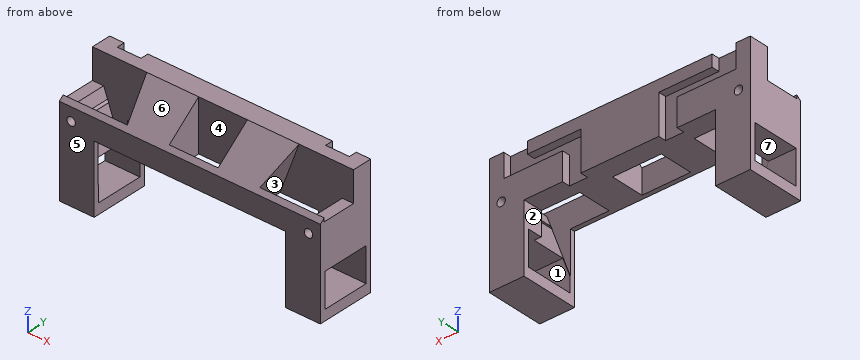
from build123d import *

# Parameters (mm, degrees)
CROQUIS1_W                  = 99
CROQUIS1_H                  = 49
SALIENTE_EXTRUIR1_DEPTH     = 22
CROQUIS2_W                  = 13
CROQUIS2_H                  = 18
CORTAR_EXTRUIR1_DEPTH       = 105.895766214
CROQUIS3_W                  = 3.5
CROQUIS3_H                  = 22
CORTAR_EXTRUIR2_DEPTH       = 105.895766214
CROQUIS4_W                  = 72.6
CROQUIS4_H                  = 26
CORTAR_EXTRUIR3_DEPTH       = 69.17620423
CORTAR_EXTRUIR4_DEPTH       = 79.584079892
CROQUIS7_W                  = 20.634922244
CROQUIS7_H                  = 12.8
CORTAR_EXTRUIR7_DEPTH       = 60
CROQUIS12_W                 = 20.6
CROQUIS12_H                 = 12.8
CORTAR_EXTRUIR8_DEPTH       = 60
CORTAR_EXTRUIR9_DEPTH       = 105.056653851
CORTAR_EXTRUIR9_DEPTH_BACK  = 105.056653851
CROQUIS16_W                 = 11.5
CROQUIS16_H                 = 12.8
CORTAR_EXTRUIR11_DEPTH      = 10
CROQUIS17_W                 = 11.5
CROQUIS17_H                 = 12.8
CORTAR_EXTRUIR12_DEPTH      = 10
CORTAR_EXTRUIR13_DEPTH      = 3
CORTAR_EXTRUIR14_DEPTH      = 69.17620423
CORTAR_EXTRUIR14_DEPTH_BACK = 69.17620423
CROQUIS20_R                 = 1.6


with BuildPart() as part:
    # Croquis1 → Saliente-Extruir1 (new body)
    with BuildSketch(Plane(origin=(0, 0, 0), x_dir=(1, 0, 0), z_dir=(0, 1, 0))):
        with Locations((10.676470588, -2.297794118)):
            Rectangle(CROQUIS1_W, CROQUIS1_H)
    extrude(amount=SALIENTE_EXTRUIR1_DEPTH)

    # Croquis2 → Cortar-Extruir1 (cut, through all)
    with BuildSketch(Plane.ZY.offset(38.823529412)):
        with Locations((-11.702205882, 11)):
            Rectangle(CROQUIS2_W, CROQUIS2_H)
    extrude(amount=-CORTAR_EXTRUIR1_DEPTH, mode=Mode.SUBTRACT)

    # Croquis3 → Cortar-Extruir2 (cut, through all)
    with BuildSketch(Plane.ZY.offset(38.823529412)):
        with Locations((25.047794118, 11)):
            Rectangle(CROQUIS3_W, CROQUIS3_H)
    extrude(amount=-CORTAR_EXTRUIR2_DEPTH, mode=Mode.SUBTRACT)

    # Croquis4 → Cortar-Extruir3 (cut, through all)
    with BuildSketch(Plane(origin=(0, 22, 0), x_dir=(1, 0, 0), z_dir=(0, 1, 0))):
        with Locations((10.676470588, 9.202205882)):
            Rectangle(CROQUIS4_W, CROQUIS4_H)
    extrude(amount=-CORTAR_EXTRUIR3_DEPTH, mode=Mode.SUBTRACT)

    # Croquis6 → Cortar-Extruir4 (cut, through all)
    with BuildSketch(Plane.XY.offset(23.297794118)):
        Polygon((19.926470588, 1.7), (19.926470588, 14.5), (1.426470588, 14.5), (1.426470588, 1.7), (10.676470588, 1.7), align=None)
    extrude(amount=-CORTAR_EXTRUIR4_DEPTH, mode=Mode.SUBTRACT)

    # Croquis7 → Cortar-Extruir7 (cut, along a direction that is not the sketch's normal)
    with BuildSketch(Plane.XY.offset(23.297794118)):
        with Locations((49.859009466, 8.1)):
            Rectangle(CROQUIS7_W, CROQUIS7_H)
    extrude(amount=-CORTAR_EXTRUIR7_DEPTH, dir=(0.346374082759158, 0, 0.9380964741393883), mode=Mode.SUBTRACT)

    # Croquis12 → Cortar-Extruir8 (cut, along a direction that is not the sketch's normal)
    with BuildSketch(Plane.XY.offset(23.297794118)):
        with Locations((-28.523529412, 8.1)):
            Rectangle(CROQUIS12_W, CROQUIS12_H)
    extrude(amount=-CORTAR_EXTRUIR8_DEPTH, dir=(-0.3463740827591596, 0, 0.9380964741393877), mode=Mode.SUBTRACT)

    # Croquis15 → Cortar-Extruir9 (cut, two sides: drawn at the far end of the back side and taken through both)
    with BuildSketch(Plane.ZY.offset(38.823529412).offset(-CORTAR_EXTRUIR9_DEPTH_BACK)):
        Polygon((23.297794118, 0), (11.797794118, 0), (23.297794118, 14.5), align=None)
    extrude(amount=CORTAR_EXTRUIR9_DEPTH + CORTAR_EXTRUIR9_DEPTH_BACK, mode=Mode.SUBTRACT)

    # Croquis16 → Cortar-Extruir11 (cut)
    with BuildSketch(Plane.ZY.offset(38.823529412)):
        with Locations((17.547794118, 8.1)):
            Rectangle(CROQUIS16_W, CROQUIS16_H)
    extrude(amount=-CORTAR_EXTRUIR11_DEPTH, mode=Mode.SUBTRACT)

    # Croquis17 → Cortar-Extruir12 (cut)
    with BuildSketch(Plane(origin=(60.176470588, 0, 0), x_dir=(0, 0, -1), z_dir=(1, 0, 0))):
        with Locations((-17.547794118, 8.1)):
            Rectangle(CROQUIS17_W, CROQUIS17_H)
    extrude(amount=-CORTAR_EXTRUIR12_DEPTH, mode=Mode.SUBTRACT)

    # Croquis18 → Cortar-Extruir13 (cut)
    with BuildSketch(Plane(origin=(0, 22, 0), x_dir=(1, 0, 0), z_dir=(0, 1, 0))):
        Polygon((-33.323529412, -23.297794118), (-24.323529412, -23.297794118), (-24.323529412, -18.818400103), (-4.120464629, -18.818400103), (-4.120464629, -3.797794118), (-11.023529412, -3.797794118), (-11.023529412, -14.307139366), (-33.323529412, -14.307139366), (-33.323529412, -18.818400103), align=None)
        Polygon((45.676470588, -18.818400103), (45.676470588, -23.297794118), (54.676470588, -23.297794118), (54.676470588, -18.818400103), (54.676470588, -14.307139366), (32.376470588, -14.307139366), (32.376470588, -3.797794118), (25.476470588, -3.797794118), (25.476470588, -18.818400103), align=None)
    extrude(amount=-CORTAR_EXTRUIR13_DEPTH, mode=Mode.SUBTRACT)

    # Croquis20 → Cortar-Extruir14 (cut, two sides: drawn at the far end of the back side and taken through both)
    with BuildSketch(Plane.XZ.offset(-CORTAR_EXTRUIR14_DEPTH_BACK)):
        with Locations(Location((-34.323529412, 6.797794118, 0), (0, 0, 270))):
            Circle(CROQUIS20_R)
        with Locations(Location((55.676470588, 6.797794118, 0), (0, 0, 270))):
            Circle(CROQUIS20_R)
    extrude(amount=CORTAR_EXTRUIR14_DEPTH + CORTAR_EXTRUIR14_DEPTH_BACK, mode=Mode.SUBTRACT)


solid = part.part
The listing builds one solid part. Answer for the finished solid, in the listing's coordinates (mm). Face numbers are marked on the shaded views. A direction names the side the tool comes from. Give positions to 0.01 mm unless a question says otherwise; leave off trailing zeros. Loops run counter-clockwise (first coordinate to the right, second up) from the corner with the lowest first, then second, coordinate; pieces in that order, holes last. Notation, with made-up numbers: (-32, 71) - (-21, 71) arc R28 cw to (-21, 103) - close; hole circle Ø10 at (-24.5, 82.5). An arc over 180 degrees is marked (long way). Write each question's results on one line, items separated by ' | '.
1. Consider probe 1 along Y at (x, z) = (54, -6.5); probe 2 along Y at (x, z) = (4, 10.5); probe 3 along X at (y, z) = (21, -9.5). Determine where each line is inside the solid, lowest interval first. Write a range as from..to.
Resolved:
probe 1: y = 0..2, 20..22 | probe 2: y = 0..1.7, 14.5..22 | probe 3: x = -38.82..-25.62, 46.98..60.18
2. Find section A-A, the plane x = 6. Write down the section's boundary in (y, z).
Resolved:
outline: (0, 3.8) - (1.7, 3.8) - (1.7, 13.15) - (0, 11.8) - close; (14.5, 3.8) - (22, 3.8) - (22, 23.3) - (14.5, 23.3) - close
3. Find section C-C, the plane y = 5. Write down the section's boundary in (x, z), then the cut area to 3 significant figures.
Resolved:
outline: (-38.82, -22.2) - (-25.62, -22.2) - (-25.62, -18.2) - (-38.82, -18.2) - close; (-38.82, -5.2) - (-28.3, -5.2) - (-32.72, 6.78) arc R1.6 cw (long way) to (-33.12, 7.85) - (-34.58, 11.8) - (-38.82, 11.8) - close; (-15.44, 15.76) - (-11.02, 3.8) - (1.43, 3.8) - (1.43, 15.76) - close; (19.93, 3.8) - (32.34, 3.8) - (36.76, 15.76) - (19.93, 15.76) - close; (46.98, -22.2) - (60.18, -22.2) - (60.18, -18.2) - (46.98, -18.2) - close; (49.65, -5.2) - (60.18, -5.2) - (60.18, 11.8) - (55.93, 11.8) - (54.47, 7.85) arc R1.6 cw (long way) to (54.08, 6.78) - close | area: 691 mm^2
4. Which of the six approach directions +Z, -Z, +X, -X, +Y, -Y give full straight-line access (tool end or side, diameter ignored) to the marked faces 1, 2, 3 and 4?
Resolved:
face 1: +X, -X | face 2: -Z, +Y, -Y | face 3: -Z | face 4: +Z, -Z
5. Find section D-D, the plane y = 16. Write down the section's boundary in (x, z).
Resolved:
outline: (-38.82, -22.2) - (-25.62, -22.2) - (-25.62, -18.2) - (-38.82, -18.2) - close; (-38.82, -5.2) - (-25.62, -5.2) - (-25.62, 3.8) - (46.98, 3.8) - (46.98, -5.2) - (60.18, -5.2) - (60.18, 23.3) - (-38.82, 23.3) - close; (46.98, -22.2) - (60.18, -22.2) - (60.18, -18.2) - (46.98, -18.2) - close; hole circle Ø3.2 at (-34.32, 6.8); hole circle Ø3.2 at (55.68, 6.8)
6. Find section B-B, the plane z = -9.5. Write down the section's boundary in (x, y), then the cut area to 3 significant figures.
Resolved:
outline: (-38.82, 0) - (-25.62, 0) - (-25.62, 1.7) - (-26.71, 1.7) - (-26.71, 2) - (-38.82, 2) - close; (-38.82, 20) - (-25.62, 20) - (-25.62, 22) - (-38.82, 22) - close; (46.98, 0) - (60.18, 0) - (60.18, 2) - (48.07, 2) - (48.07, 1.7) - (46.98, 1.7) - close; (46.98, 20) - (60.18, 20) - (60.18, 22) - (46.98, 22) - close | area: 105 mm^2
7. Flat-ended cylindrical pins translate along their axes: P1, Ø2.5, axis at x = 35.5, y = 20, coming from the -Z side; P2, Ø10, axis at y = 10.5, z = 12.5, coming from the -X side; P3, Ø2.5, axis at x = -27, y = 20.5, coming from the +Z side; P4, Ø4.5, axis at x = 58.5, y = 5.5, coming from the +Z side. Find the tip coordinate at first contact, or state that the pin passes through.
Resolved:
P1: stops at z = 3.8 | P2: stops at x = -38.82 | P3: stops at z = 14.31 | P4: stops at z = 11.8
8. For a pull along Z with two mould halves and no side action, classify the marked faces 5, 6 and 7 as +Z half, -Z half, draft (parallel to the pull), parting line (faces both ways), or undercut.
Resolved:
face 5: draft | face 6: +Z half | face 7: undercut
